Input: dimensioned drawing with shaded views. Units: mm. Origin: part minimum x, y, z. A direction names the side the tool comes from. Give positions to 0.01 mm unless a question says otherwise; leave off trailing zeros. Write each loop counter-clockwise with the first axis right and the second up, starting at its lowest first coordinate (ties: lowest second). Pieces come first, ordered by that corner, then holes.
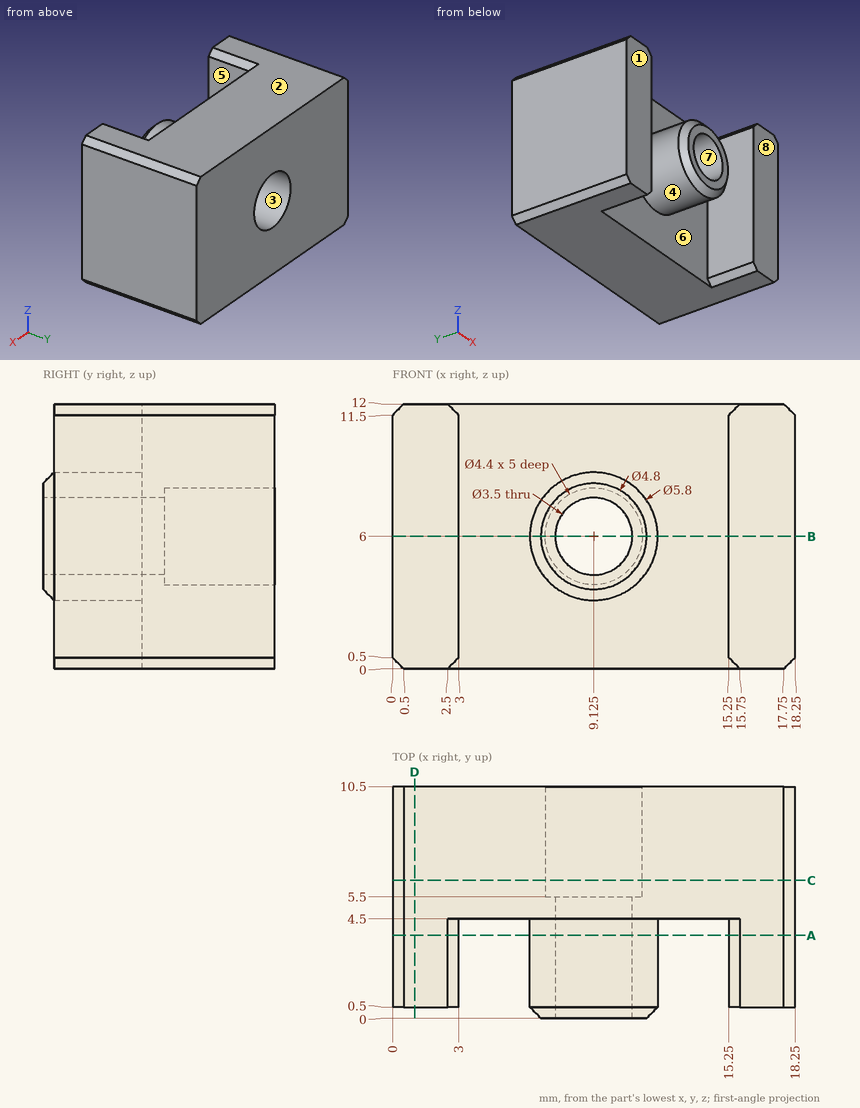
Item 1: Section D-D, the plane x = 1. Return the cut outline in (y, z), plus the area to 3 significant figures.
Found:
outline: (0.5, 0) - (10.5, 0) - (10.5, 12) - (0.5, 12) - close
area: 120 mm2
Item 2: Section A-A, the plane y = 3.75. Return the cut outline in (x, z) (3 decimals), plus the area to 3 significant figures.
Found:
outline: (0, 0.5) - (0.5, 0) - (2.5, 0) - (3, 0.5) - (3, 11.5) - (2.5, 12) - (0.5, 12) - (0, 11.5) - close; circle Ø5.8 at (9.125, 6); (15.25, 0.5) - (15.75, 0) - (17.75, 0) - (18.25, 0.5) - (18.25, 11.5) - (17.75, 12) - (15.75, 12) - (15.25, 11.5) - close; hole circle Ø3.5 at (9.125, 6)
area: 87.8 mm2
Item 3: Pin query (flat end, axial travel): pin 1 Ø3.5 at (x, z) = (17.5, 5.5) entering from -Y. Return the tip coordinate at first contact, or that it passes through.
Found:
pin 1: stops at y = 0.5
Item 4: Line query: L1, parallel to Y at x = 17.5, z = 7; L2, parallel to X at y = 4, z = 4.75; L3, parallel to Y at x = 14.5, z = 1.5. Output: solid intervals per line, ascending.
Found:
L1: y = 0.5 to 10.5
L2: x = 0 to 3, 6.51 to 7.9, 10.35 to 11.74, 15.25 to 18.25
L3: y = 4.5 to 10.5
Item 5: Reachability of the marked faces 5, 6, 7 and 8 from +Z, -Z, +X, -X, +Y, -Y: full face, straight path, thin tool, end or side. Return the list, or none.
Found:
face 5: +Z, -Z, -Y
face 6: -Y
face 7: +Y, -Y
face 8: +Z, -Z, +X, -Y
Item 6: Section B-B, the plane z = 6. Return the cut outline in (x, y) (3 decimals), plus the area to 3 significant figures.
Found:
outline: (0, 0.5) - (3, 0.5) - (3, 4.5) - (6.225, 4.5) - (6.225, 0.5) - (6.725, 0) - (7.375, 0) - (7.375, 5.5) - (6.925, 5.5) - (6.925, 10.5) - (0, 10.5) - close; (10.875, 0) - (11.525, 0) - (12.025, 0.5) - (12.025, 4.5) - (15.25, 4.5) - (15.25, 0.5) - (18.25, 0.5) - (18.25, 10.5) - (11.325, 10.5) - (11.325, 5.5) - (10.875, 5.5) - close
area: 118 mm2
Item 7: Pull-direction query (Z, two-part tool) for the marked faces 1, 2, 3 and 4; classes: +Z half, -Z half, draft (parallel to the pull), parting line (faces both ways), or undercut.
Found:
face 1: draft
face 2: +Z half
face 3: undercut
face 4: parting line
Item 8: Section C-C, the plane y = 6.25. Return the cut outline in (x, z) (3 decimals), plus the area to 3 significant figures.
Found:
outline: (0, 0.5) - (0.5, 0) - (17.75, 0) - (18.25, 0.5) - (18.25, 11.5) - (17.75, 12) - (0.5, 12) - (0, 11.5) - close; hole circle Ø4.4 at (9.125, 6)
area: 203 mm2
